Autodesk Inventor part; units mm, degrees
ref_plane "YZ Plane" through (0, 0, 0) normal (1, 0, 0) x (0, 1, 0)
ref_plane "XZ Plane" through (0, 0, 0) normal (0, 1, 0) x (-1, 0, 0)
ref_plane "XY Plane" through (0, 0, 0) normal (0, 0, 1) x (1, 0, 0)
ref_plane "Work Plane1" through (-22, 18, -9.9035) normal (0, -1, 0) x (0, 0, -1)
sketch "Sketch1" plane through (-22, 18, -9.9035) normal (0, -1, 0) x (0, 0, -1)
  spline S0 degree 3 poles (41.079, 4.2882) (41.1539, 4.1612) (41.2485, 4.0469) (41.4813, 3.8418) (41.6216, 3.7561) (41.9369, 3.6326) (42.1108, 3.5998) (42.4706, 3.6003) (42.653, 3.6369) (42.99, 3.7773) (43.142, 3.8786) (43.3765, 4.1113) (43.4651, 4.2329) (43.6017, 4.5018) (43.648, 4.6478) (43.6753, 4.8356) (43.6793, 4.8732) (43.683, 4.9311) (43.6838, 4.9515) (43.6846, 4.9887) (43.6846, 5.0055) (43.684, 5.0419) (43.6833, 5.0615) (43.6802, 5.1152) (43.6769, 5.1493) (43.6596, 5.2804) (43.6366, 5.3761) (43.5593, 5.5938) (43.4972, 5.7121) (43.331, 5.9422) (43.2234, 6.0494) (42.9677, 6.2329) (42.819, 6.3043) (42.4931, 6.3953) (42.3177, 6.4104) (41.96, 6.3744) (41.7817, 6.3196) (41.4606, 6.1462) (41.3201, 6.0307) (41.1088, 5.775) (41.0318, 5.6432) (40.9361, 5.3938) (40.9083, 5.2815) (40.8908, 5.1364) (40.8882, 5.1057) (40.8856, 5.0572) (40.8849, 5.0395) (40.8844, 5.0069) (40.8844, 4.9919) (40.885, 4.9591) (40.8856, 4.9412) (40.8884, 4.891) (40.8913, 4.8587) (40.9067, 4.735) (40.9271, 4.645) (40.9875, 4.4636) (41.0287, 4.3733) (41.079, 4.2882) knots 0 0 0 0 0.044326 0.044326 0.093383 0.093383 0.146079 0.146079 0.201356 0.201356 0.255644 0.255644 0.300529 0.300529 0.346168 0.346168 0.357482 0.357482 0.363591 0.363591 0.368644 0.368644 0.374518 0.374518 0.384776 0.384776 0.41421 0.41421 0.454101 0.454101 0.499414 0.499414 0.548537 0.548537 0.600928 0.600928 0.656444 0.656444 0.710644 0.710644 0.75624 0.75624 0.790854 0.790854 0.800101 0.800101 0.805408 0.805408 0.809903 0.809903 0.81526 0.81526 0.824988 0.824988 0.852648 0.852648 0.88238 0.88238 0.88238 0.88238
  point P0 (-9.9035, 22)
  point P1 (41.079, 4.2882)
extrude "Extrusion1" add sketch "Sketch1" against normal blind 24.6
sketch "Sketch2" plane through (-17, 42.6, -52.188) normal (0, 1, 0) x (1, 0, 0)
  circle A0 centre (0, 0) radius 2.95
  point P0 (17, -52.188)
  dimension "d2" = 5.9
extrude "Extrusion2" add sketch "Sketch2" along normal blind 2.4
chamfer "Chamfer1" distance 2 angle 30 1 edges at (-19.95, 45, -52.188) measured on face at (-16.264, 45, -53.3107)
properties part number "longerScrew"
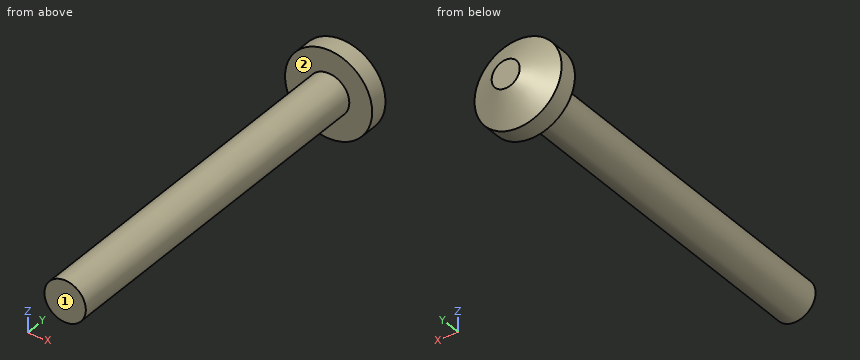
Here's how the part is built. I have some questions about the finished solid (model axes, mm). Face numbers are marked on the shaded views. A direction names the side the tool comes from. Coordinates: 2 decimals unless noted, no trailing zeros. Use a Markdown table: item, result. Add a question column.
(1) I'm going to push flat-ended pins straight in: P1, Ø1.5, axis at y = 22.5, z = -52, coming from the -X side; P2, Ø2, axis at x = -15.5, y = 41, coming from the -Z side; P3, Ø1.5, axis at y = 32.5, z = -52.5, coming from the +X side. Where does each tip first touch, or does it pass through?
(2) Please list where these lines run through material, in increasing order: line 1 (Z direction, x = -16.95, y = 31.75); line 2 (X direction, y = 19.75, z = -52.7); line 3 (X direction, y = 31.75, z = -51.5).
(3) For the marked faces 1 and 2, which set-ups out of +Z, -Z, +X, -X, +Y, -Y let a thin tool reach every point of the face, with its end or its side?
Outcome:
| question | item | result |
|---|---|---|
| 1 | P1 | stops at x = -18.4 |
| 1 | P2 | stops at z = -53.5 |
| 1 | P3 | stops at x = -15.6 |
| 2 | line 1 | z = -53.59 to -50.79 |
| 2 | line 2 | x = -18.3 to -15.7 |
| 2 | line 3 | x = -18.22 to -15.78 |
| 3 | face 1 | +Z, -Z, +X, -X, -Y |
| 3 | face 2 | -Y |
